Source: three-view drawing plus pictorial views. Frame: mm from the lowest corner of the part. A direction names the side the tool comes from. Round coordinates to 2 decimals unless told otherwise and drop trailing zeros. Loops run counter-clockwise (first coordinate to the right, second up) from the corner with the lowest first, then second, coordinate; pieces in that order, holes last. Notation, with made-up numbers: (88, 87.25) -> (105, 87.25) arc R22 ccw to (105, 122.25) -> close; hole circle Ø10 at (27.5, 60.5). An arc over 180 degrees is marked (long way). Answer in a Markdown table with one row per item.
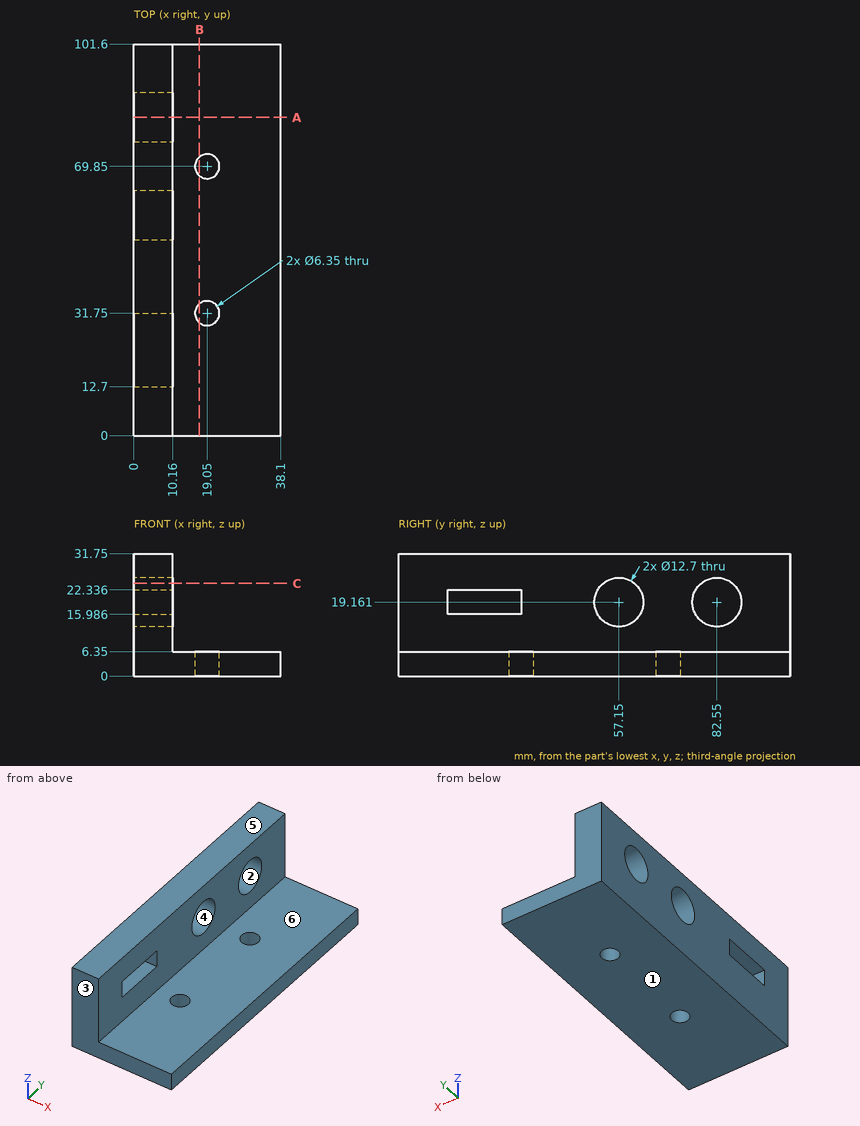
Item 1: Draft query along Y for the marked faces 1, 2, 3 and 4. Return one class per face: pulls with the +Y half, pulls with the -Y half, needs draft (parallel to the pull), parting line crosses it, or undercut.
Answer:
| item | result |
|---|---|
| face 1 | needs draft |
| face 2 | undercut |
| face 3 | pulls with the -Y half |
| face 4 | undercut |
Item 2: Pin query (flat end, axial travel): pin 1 Ø11.5 at (y, z) = (82.55, 19.16) entering from +X; pin 2 Ø22.5 at (x, y) = (22.5, 56.5) entering from +Z. Return the tip coordinate at first contact, or that it passes through.
Answer:
| item | result |
|---|---|
| pin 1 | passes through |
| pin 2 | stops at z = 6.35 |
Item 3: Cut plane A-A (y = 82.55). Output: boundary loops of the cut face in (x, z), then the cut area to 3 significant figures.
Answer:
| item | result |
|---|---|
| outline | (0, 0) -> (38.1, 0) -> (38.1, 6.35) -> (10.16, 6.35) -> (10.16, 12.81) -> (0, 12.81) -> close; (0, 25.51) -> (10.16, 25.51) -> (10.16, 31.75) -> (0, 31.75) -> close |
| area | 371 mm² |
Item 4: Cut plane B-B (x = 17). Count the separate pieces of the cut face and the enclosed holes in it.
Answer:
| item | result |
|---|---|
| separate pieces | 3 |
| enclosed holes | 0 |
Item 5: Line query: probe 1 along Y at (x, z) = (19, 2) (1 decimal); probe 2 along Y at (x, z) = (9.5, 19); probe 3 along Y at (x, z) = (9, 24). Output: solid intervals per line, ascending. Write a range as [from, to].
Answer:
| item | result |
|---|---|
| probe 1 | y = [0, 28.6], [34.9, 66.7], [73, 101.6] |
| probe 2 | y = [0, 12.7], [31.75, 50.8], [63.5, 76.2], [88.9, 101.6] |
| probe 3 | y = [0, 53.04], [61.26, 78.44], [86.66, 101.6] |
Item 6: Reachability of the marked faces 5 and 6 from +Z, -Z, +X, -X, +Y, -Y: full face, straight path, thin tool, end or side. Return the list, or none.
Answer:
| item | result |
|---|---|
| face 5 | +Z, +X, -X, +Y, -Y |
| face 6 | +Z, +X, +Y, -Y |
Item 7: Cut plane C-C (z = 24). Output: boundary loops of the cut face in (x, y).
Answer:
| item | result |
|---|---|
| outline | (0, 0) -> (10.16, 0) -> (10.16, 53.04) -> (0, 53.04) -> close; (0, 61.26) -> (10.16, 61.26) -> (10.16, 78.44) -> (0, 78.44) -> close; (0, 86.66) -> (10.16, 86.66) -> (10.16, 101.6) -> (0, 101.6) -> close |
